Can you work these out from the model? Positions are in its coordinate system, mm. Face numbers are marked on the shaded views. A direction names the side the tool comes from. Coordinates: 2 decimals unless noted, no trailing zeros. Loops run counter-clockwise (first coordinate to the right, second up) from the corner with the lowest first, then second, coordinate; pieces in that order, holes last. Notation, with made-up numbers: M 88,4.25 L 141,4.25 A9 ccw 141,13.25 Z; hole C -29,63.5 d8. An arc over 180 degrees is marked long. Answer as a JSON object with one key per item and string values. Group by question number.
Item 1: Suppose I cut it at D-D (z = 12). Count the separate pieces of the cut face and the enclosed holes in it, then the cut area to 3 significant figures.
Item 2: Which directions (+Z, -Z, +X, -X, +Y, -Y) give clear straight access to the entire face, cutting with the end or side of a thin tool? Please do the marked faces 1 and 2.
Item 3: I'm going to push flat-ended pins straight in: pin 1 Ø3 at (x, z) = (-72.5, 16) entering from -Y; pin 2 Ø5 at (x, z) = (74.5, 26) entering from -Y; pin 3 Ø1.8 at (y, z) = (49, 24) entering from +X; pin 4 Ø5.5 at (x, y) = (70, -45) entering from +Z. Where does each tip first touch, or does it pass through?
Item 4: Suppose I cut it at A-A (x = -41.5). Write out the boundary of the cut face in (y, z).
Item 5: Suppose I cut it at C-C (y = 26). Write out the boundary of the cut face in (x, z).
Item 6: We'd pull the mould along X, two halves only. Please class the marked faces 3, 4 and 5: +X half, -X half, draft (parallel to the pull), parting line (faces both ways), or undercut.
Item 7: If I drill on line 1 (Y direction, x = -70, z = 43); line 2 (X direction, y = -11.5, z = 46.5); line 3 (Y direction, x = 49.5, z = 6.5), over which ranges is the centre line in solid material (lowest first)?
Item 8: Suppose I cut it at B-B (z = 54). Write out the boundary of the cut face in (x, y), then the cut area to 3 significant figures.
```python
from build123d import *

# Parameters (mm, degrees)
SKETCH_1_R             = 4.75
EXTRUDE_1_DEPTH        = 58
CUT_EXTRUDE_1_DEPTH    = 169
PATTERN_LINEAR_1_COUNT = 6
PATTERN_LINEAR_1_PITCH = 10


with BuildPart() as part:
    # Эскиз1 → Бобышка-Вытянуть1 (new body)
    with BuildSketch(Plane.XY):
        with BuildLine():
            Line((-70, 55), (70, 55))
            ThreePointArc((70, 55), (77.071067812, 52.071067812), (80, 45))
            Line((80, 45), (80, -45))
            ThreePointArc((80, -45), (77.071067812, -52.071067812), (70, -55))
            Line((70, -55), (-70, -55))
            ThreePointArc((-70, -55), (-77.071067812, -52.071067812), (-80, -45))
            Line((-80, -45), (-80, 45))
            ThreePointArc((-80, 45), (-77.071067812, 52.071067812), (-70, 55))
        make_face()
        with Locations((70, 45)):
            Circle(SKETCH_1_R, mode=Mode.SUBTRACT)
        with Locations((70, -45)):
            Circle(SKETCH_1_R, mode=Mode.SUBTRACT)
        with Locations((-70, -45)):
            Circle(SKETCH_1_R, mode=Mode.SUBTRACT)
        with Locations((-70, 45)):
            Circle(SKETCH_1_R, mode=Mode.SUBTRACT)
        with BuildLine():
            Line((-64, 51), (64, 51))
            Line((64, 51), (64, 45))
            ThreePointArc((64, 45), (65.757359313, 40.757359313), (70, 39))
            Line((70, 39), (76, 39))
            Line((76, 39), (76, -39))
            Line((76, -39), (70, -39))
            ThreePointArc((70, -39), (65.757359313, -40.757359313), (64, -45))
            Line((64, -45), (64, -51))
            Line((64, -51), (-64, -51))
            Line((-64, -51), (-64, -45))
            ThreePointArc((-64, -45), (-65.757359313, -40.757359313), (-70, -39))
            Line((-70, -39), (-76, -39))
            Line((-76, -39), (-76, 39))
            Line((-76, 39), (-70, 39))
            ThreePointArc((-70, 39), (-65.757359313, 40.757359313), (-64, 45))
            Line((-64, 45), (-64, 51))
        make_face(mode=Mode.SUBTRACT)
    extrude(amount=EXTRUDE_1_DEPTH)

    # Эскиз2 → Вырез-Вытянуть1 (cut)
    with BuildSketch(Plane.ZY.offset(80)):
        with BuildLine():
            Line((46.937976774, 15.864192118), (8.050346324, 33.995467526))
            ThreePointArc((8.050346324, 33.995467526), (5.329053146, 33.235382363), (5.916242197, 30.471621333))
            Line((5.916242197, 30.471621333), (45.193454902, 12.123052891))
            ThreePointArc((45.193454902, 12.123052891), (47.936328276, 13.121453414), (46.937976774, 15.864192118))
        make_face()
    cut_extrude_1 = extrude(amount=-CUT_EXTRUDE_1_DEPTH, mode=Mode.SUBTRACT)

    # Линейный массив1: Вырез-Вытянуть1 ×6
    with Locations(*[(0, -i * PATTERN_LINEAR_1_PITCH, 0) for i in range(1, PATTERN_LINEAR_1_COUNT)]):
        add(cut_extrude_1, mode=Mode.SUBTRACT)


solid = part.part
```
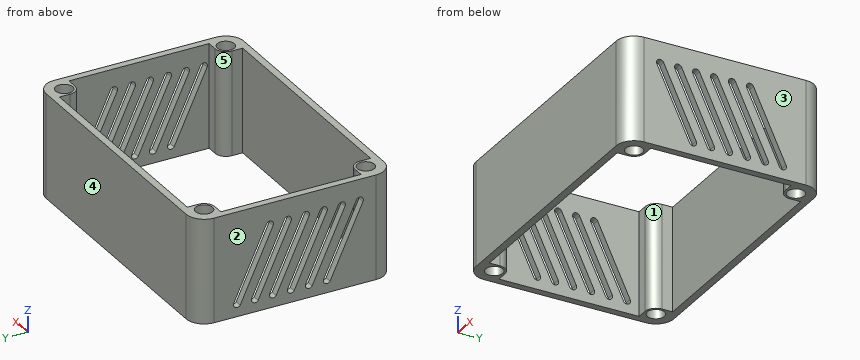
From the geometry:
{
 "1": {"separate pieces": "12", "enclosed holes": "4", "area": "2,050 mm2"},
 "2": {"face 1": "+Z, -Z", "face 2": "+Z, -Z, -X, +Y, -Y"},
 "3": {"pin 1": "y = -54.95", "pin 2": "y = -54.8", "pin 3": "x = 79.51", "pin 4": "through"},
 "4": {"outline": "M -55,0 L -51,0 L -51,58 L -55,58 Z; M 51,0 L 55,0 L 55,58 L 51,58 Z"},
 "5": {"outline": "M -80,0 L -76,0 L -76,15.49 L -80,15.49 Z; M -80,25.2 L -76,25.2 L -76,58 L -80,58 Z; M 76,0 L 80,0 L 80,15.49 L 76,15.49 Z; M 76,25.2 L 80,25.2 L 80,58 L 76,58 Z"},
 "6": {"face 3": "+X half", "face 4": "draft", "face 5": "undercut"},
 "7": {"line 1": "-55 to -49.75, -40.25 to -39, 39 to 40.25, 49.75 to 55", "line 2": "-80 to -76, 76 to 80", "line 3": "-55 to -51, 51 to 55"},
 "8": {"outline": "M -80,-45 A10 ccw -70,-55 L 70,-55 A10 ccw 80,-45 L 80,45 A10 ccw 70,55 L -70,55 A10 ccw -80,45 Z; hole M -76,-39 L -70,-39 A6 cw -64,-45 L -64,-51 L 64,-51 L 64,-45 A6 cw 70,-39 L 76,-39 L 76,39 L 70,39 A6 cw 64,45 L 64,51 L -64,51 L -64,45 A6 cw -70,39 L -76,39 Z; hole C -70,-45 d9.5; hole C -70,45 d9.5; hole C 70,-45 d9.5; hole C 70,45 d9.5", "area": "2,270 mm2"}
}
